For this review, take the finished solid that the model builds, in its own axes (mm). A direction names the side the tool comes from. Give positions to 0.01 mm unless a question says otherwise; leave off trailing zeros. Order: outer loops, then holes, each group sorted by start corner. A loop starts at its lowest first (then second) coordinate and runs counter-clockwise, first axis right, second up. Notation, with made-up numbers: M 27.5,-10 L 55.5,-10 A16 cw 55.5,6 Z; hole C -35,14 d1. An arc over 180 degrees is marked long. Answer as CSV lines item,"result". Start each with the question number.
1. Mouldability with a two-part tool opening along X and no side actions: class faces 4 (the flat face through (15.23, 183, 39)), 5 (the flat face through (17.9, 136.85, -3.96)), 6 (the flat face through (-19.09, 179.94, 33.47)), 7 (the flat face through (18.992, 155.348, 25.4)) as pulls with the +X half, pulls with the -X half, needs draft (parallel to the pull), parting line crosses it, or undercut.
2. We need section B-B, the plane y = 114. Give the boundary of the cut face in (x, z), and give its area (3 significant figures).
3. We need section A-A, the plane x = 18.5. Give the boundary of the cut face in (y, z).
4. For line 1 along Z through (x, y) = (-6.5, 175); line 2 along Z through (x, y) = (-3.5, 111.5); line 3 along Y through (x, z) = (-2, 34), list the stretches that pass through material, from the lowest coordinate up.
5. Machinability: for faces 1 (the flat face through (-19.709, 135.845, -5.455)), 2 (the flat face through (-15.23, 183, 39)), 3 (the flat face through (-5.4, 172.73, 52.52)), which of the approach directions +Z, -Z, +X, -X, +Y, -Y give a long, thin tool a straight path to every point of the face, cutting with its end or side? Answer none if there is none.
6. Clearance check with flat-ended pins moving along their axes: P1, Ø2, axis at x = 1, z = -5.5, coming from the -Y side; P2, Ø6, axis at y = 121.5, z = -32.5, coming from the -X side; P3, Ø3, axis at x = 4.5, z = -39, coming from the -Y side; P4, Ø2.5, axis at y = 186.83, z = 36.76, coming from the -X side (3 decimals). State where each tip first meets the part, or that it passes through.
7. We need section C-C, the plane x = -12.5. Give the boundary of the cut face in (y, z).
from build123d import *

# Parameters (mm, degrees)
BOSS_EXTRUDE1_DEPTH = 8.89
SKETCH9_W           = 38.1
SKETCH9_H           = 170.494756514
CUT_EXTRUDE1_DEPTH  = 10.16
BOSS_EXTRUDE2_DEPTH = 63.5
SKETCH12_W          = 7.62
SKETCH12_H          = 12.7
BOSS_EXTRUDE3_DEPTH = 25.4
SKETCH13_R          = 2.031999997
CUT_EXTRUDE2_DEPTH  = 46.699791471


with BuildPart() as part:
    # Sketch2 → Boss-Extrude1 (new body)
    with BuildSketch(Plane(origin=(0, 107.565160262, -63.883098153), x_dir=(1, 0, 0), z_dir=(0, -0.859797598, 0.510634988))):
        Polygon((-16.72668145, 3.22686704), (-22.849895735, 69.859735371), (22.849895735, 69.859735371), (16.72668145, 3.22686704), align=None)
    extrude(amount=BOSS_EXTRUDE1_DEPTH)

    # Sketch9 → Cut-Extrude1 (cut)
    with BuildSketch(Plane(origin=(52.068196995, 40.765068024, -18.64540373), x_dir=(0.369989021, -0.048221617, 0.927783811), z_dir=(-0.75783864, -0.59332463, 0.27137885))):
        with Locations((0.146468301, 41.148554402)):
            Rectangle(SKETCH9_W, SKETCH9_H)
    cut_extrude1 = extrude(amount=CUT_EXTRUDE1_DEPTH, mode=Mode.SUBTRACT)

    # Mirror1: Cut-Extrude1 across plane
    add(cut_extrude1.mirror(Plane.ZY), mode=Mode.SUBTRACT)

    # Sketch11 → Boss-Extrude2 (add)
    with BuildSketch(Plane(origin=(0, 35.672825136, 60.065232647), x_dir=(1, 0, 0), z_dir=(0, 0.510634988, 0.859797598))):
        Polygon((-22.849895735, 125.105211449), (-15.24, 116.215211449), (15.24, 116.215211449), (22.849895735, 125.105211449), align=None)
    extrude(amount=BOSS_EXTRUDE2_DEPTH)

    # Sketch12 → Boss-Extrude3 (add)
    with BuildSketch(Plane(origin=(0, 107.565160262, -63.883098153), x_dir=(-1, 0, 0), z_dir=(0, 0.859797598, -0.510634988))):
        with Locations((-19.039895735, 127.009735371)):
            Rectangle(SKETCH12_W, SKETCH12_H)
    boss_extrude3 = extrude(amount=BOSS_EXTRUDE3_DEPTH)

    # Mirror2: Boss-Extrude3 across plane
    add(boss_extrude3.mirror(Plane(origin=(0, 0, 0), x_dir=(0, 0, 1), z_dir=(1, 0, 0))))

    # Sketch13 → Cut-Extrude2 (cut, through all)
    with BuildSketch(Plane.ZY.offset(22.849895735)):
        with Locations((36.759282263, 186.834421892)):
            Circle(SKETCH13_R)
    extrude(amount=-CUT_EXTRUDE2_DEPTH, mode=Mode.SUBTRACT)


solid = part.part
Result set:
1,face 4,"undercut"
1,face 5,"undercut"
1,face 6,"needs draft"
1,face 7,"pulls with the +X half"
2,outline,"M -18.96,-35.64 L -17.59,-53.05 L 17.59,-53.05 L 18.96,-35.64 Z"
2,area,"636 mm2"
3,outline,"M 111.42,-39.98 L 119.07,-44.52 L 169.18,39.86 L 191.02,26.89 L 197.5,37.81 L 171.29,53.37 L 138.87,-1.22 L 136.73,-5.89 L 131.51,-6.16 Z; hole C 186.83,36.76 d4.06"
4,line 1,"49.66 to 51.17"
4,line 2,"-57.26 to -39.85"
4,line 3,"155.36 to 165.7"
5,face 1,"+Z, -Y"
5,face 2,"-Z, +Y"
5,face 3,"+Z, +X, -X, +Y"
6,P1,"y = 131.31"
6,P2,"x = -19.84"
6,P3,"y = 111.11"
6,P4,"through"
7,outline,"M 101.57,-56.57 L 109.21,-61.11 L 175.66,50.78 L 168.02,55.32 Z"
